Verification items for the finished model (mm, model axes). A direction names the side the tool comes from. Give positions to 0.01 mm unless a question says otherwise; leave off trailing zeros. Write each loop counter-clockwise with the first axis right and the second up, starting at its lowest first coordinate (ties: lowest second). Pieces come first, ordered by that corner, then holes. Notation, with made-up numbers: M 23.25,29 L 62.25,29 A8 cw 62.25,42 Z; hole C 69,-13.5 d3. An arc over 180 degrees is marked long. Answer as a JSON object with one key per item and string values.
```python
from build123d import *

# Parameters (mm, degrees)
SKETCH2_W           = 8
SKETCH2_H           = 30
BOSS_EXTRUDE1_DEPTH = 4
CUT_EXTRUDE1_DEPTH  = 5
SKETCH4_W           = 8
SKETCH4_H           = 8
BOSS_EXTRUDE2_DEPTH = 20
SKETCH5_R           = 3.3
CUT_EXTRUDE2_DEPTH  = 15.5
CUT_EXTRUDE3_REACH  = 10


with BuildPart() as part:
    # Sketch2 → Boss-Extrude1 (new body)
    with BuildSketch(Plane(origin=(0, 0, 0), x_dir=(1, 0, 0), z_dir=(0, 1, 0))):
        Rectangle(SKETCH2_W, SKETCH2_H)
    extrude(amount=BOSS_EXTRUDE1_DEPTH)

    # Sketch3 → Cut-Extrude1 (cut, through all)
    with BuildSketch(Plane(origin=(0, 0, 0), x_dir=(1, 0, 0), z_dir=(0, 1, 0))):
        with BuildLine():
            Line((-2, -11.5), (-2, 11.5))
            ThreePointArc((-2, 11.5), (0, 13.5), (2, 11.5))
            Line((2, 11.5), (2, -11.5))
            ThreePointArc((2, -11.5), (0, -13.5), (-2, -11.5))
        make_face()
    extrude(amount=CUT_EXTRUDE1_DEPTH, mode=Mode.SUBTRACT)

    # Sketch4 → Boss-Extrude2 (add)
    with BuildSketch(Plane(origin=(0, 0, 0), x_dir=(1, 0, 0), z_dir=(0, 1, 0))):
        with Locations((0, -19)):
            Rectangle(SKETCH4_W, SKETCH4_H)
    extrude(amount=BOSS_EXTRUDE2_DEPTH)

    # Sketch5 → Cut-Extrude2 (cut)
    with BuildSketch(Plane(origin=(0, 20, 0), x_dir=(1, 0, 0), z_dir=(0, 1, 0))):
        with Locations((0, -19)):
            Circle(SKETCH5_R)
    extrude(amount=-CUT_EXTRUDE2_DEPTH, mode=Mode.SUBTRACT)

    # Sketch6 → Cut-Extrude3 (cut, up to next)
    with BuildSketch(Plane.ZY.offset(4), mode=Mode.PRIVATE) as cut_extrude3_sk1:
        with BuildLine():
            Line((19.5, 4.5), (18.5, 4.5))
            ThreePointArc((18.5, 4.5), (17, 6), (18.5, 7.5))
            Line((18.5, 7.5), (19.5, 7.5))
            ThreePointArc((19.5, 7.5), (21, 6), (19.5, 4.5))
        make_face()
    cut_extrude3_tool1 = extrude(cut_extrude3_sk1.sketch, amount=-CUT_EXTRUDE3_REACH, mode=Mode.PRIVATE) & part.part
    add(cut_extrude3_tool1.solids().sort_by_distance((-4, 6, 19))[0], mode=Mode.SUBTRACT)


solid = part.part
```
1) Section check A-A on z = -1. Record the boundary of the cut face in (x, y).
Completed:
{"outline": "M -4,0 L -2,0 L -2,4 L -4,4 Z; M 2,0 L 4,0 L 4,4 L 2,4 Z"}
2) Go/stop test with flat-tipped pins: pin 1 (0.8 mm diameter, centred on x = -4, z = 19, fed in from -Y); pin 2 (2 mm diameter, centred on x = -2, z = 19, fed in from +Y); pin 3 (4 mm diameter, centred on x = 0.5, z = -0.5, fed in from +Y). Record where each tip stops, or that it passes through.
Completed:
{"pin 1": "stops at y = 0", "pin 2": "stops at y = 4.5", "pin 3": "stops at y = 4"}
3) Thickness scan on L1, parallel to X at y = 14.25, z = 19; L2, parallel to Z at x = -0.25, y = 13; L3, parallel to Y at x = 2.5, z = -9. Record the ranges inside material, lowest first.
Completed:
{"L1": "x = -4 to -3.3, 3.3 to 4", "L2": "z = 15 to 15.71, 22.29 to 23", "L3": "y = 0 to 4"}
4) Access from +Z, -Z, +X, -X, +Y, -Y to the whole of each face (thin tool, end or side, straight path). Record for faces 4 (the face through (2, 2, 0)), 5 (the face through (-3, 6, 17)), 6 (the face through (-4, 3, 13)), 7 (the face through (-3, 4, 0)), 8 (the face through (3.05, 12.36, 20.26)).
Completed:
{"face 4": "+Y, -Y", "face 5": "-X", "face 6": "+Z, -Z, -X, +Y, -Y", "face 7": "-Z, +X, -X, +Y", "face 8": "+Y"}
5) Section check C-C on y = 6. Record the boundary of the cut face in (x, z).
Completed:
{"outline": "M -4,15 L 4,15 L 4,23 L -4,23 L -4,21 L -2.62,21 A3.3 cw long -2.62,17 L -4,17 Z"}
6) Section check B-B on x = 0. Record the boundary of the cut face in (y, z), and give its area (3 significant figures).
Completed:
{"outline": "M 0,-15 L 4,-15 L 4,-13.5 L 0,-13.5 Z; M 0,13.5 L 4,13.5 L 4,15 L 20,15 L 20,15.7 L 4.5,15.7 L 4.5,22.3 L 20,22.3 L 20,23 L 0,23 Z", "area": "69.7 mm2"}
7) Release check for a two-part mould opening along Z. For faces 1 (the face through (-3, 0, 8)), 2 (the face through (-3, 6, 21)), 3 (the face through (0, 12, 15)) record: pulls with the +Z half, pulls with the -Z half, needs draft (parallel to the pull), parting line crosses it, or undercut.
Completed:
{"face 1": "needs draft", "face 2": "undercut", "face 3": "pulls with the -Z half"}
8) Section check D-D on y = 8.75. Record the boundary of the cut face in (x, z).
Completed:
{"outline": "M -4,15 L 4,15 L 4,23 L -4,23 Z; hole C 0,19 d6.6"}
